from build123d import *

# Parameters (mm, degrees)
F1_DEPTH = 25.4
F2_R     = 28.1548982212
F3_DEPTH = 25.401
F4_R     = 12.69999


# Not quite as in the source:
# - a fillet or chamfer is up to 0.001 mm smaller than in the source, because OpenCascade refuses the exact size


with BuildPart() as f1:
    # F0 (on Front) → F1 (new body)
    with BuildSketch(Plane.XZ):
        Polygon((0, 63.7160863788), (0, 0), (254, 0), (254, 177.8), (221.1352040053, 177.8), (221.1352040053, 63.7160863788), (125.8798138147, 63.7160863788), (125.8798138147, 177.8), align=None)
    extrude(amount=F1_DEPTH)

    # F2 (on face) → F3 (cut, through all)
    with BuildSketch(Plane(origin=(0, 0, 0), x_dir=(-1, 0, 0), z_dir=(0, 1, 0))):
        with Locations((-74.7735798359, 45.1450571418)):
            Circle(F2_R)
    extrude(amount=-F3_DEPTH, mode=Mode.SUBTRACT)

    # F4 (radius 12.7 in the source; OpenCascade refuses exactly that, so slightly less here)
    f4_edges = [f1.edges().sort_by_distance(p)[0] for p in [
        (102.928478, 0, 45.145057),
        (102.928478, -25.4, 45.145057),
    ]]
    fillet(f4_edges, radius=F4_R)


solid = f1.part
CAD build for the part. Positions are in the model's coordinates, mm. A direction names the side the tool comes from. Round coordinates to 2 decimals unless told otherwise and drop trailing zeros. Loops run counter-clockwise (first coordinate to the right, second up) from the corner with the lowest first, then second, coordinate; pieces in that order, holes last.
(1) Cut at A-A (z = 102). Give the cut face in (x, y).
(2) Drop flat-ended pins along their axis: pin 1 (1 mm diameter, centred on x = 129.5, y = -20.5, fed in from +Z); pin 2 (1 mm diameter, centred on y = -14, z = 149, fed in from -X); pin 3 (10 mm diameter, centred on x = 35, y = -16.5, fed in from +Z). Give the stop position or say it passes through.
(3) Two-plate mould, pull along X, no slides. Class faces 3 (the flat face through (254, -13, 88)), 4 (the flat face through (174, -13, 63.716)), 5 (the flat face through (125, 0, 70)), 6 (the flat face through (221.135, -13, 122)): +X half, -X half, draft (parallel to the pull), parting line (faces both ways), or undercut.
(4) Cut at D-D (z = 127). Give the cut face in (x, y).
(5) Wall check: line 1 along X through (y, z) = (-4, 72.5); line 2 along Z through (x, y) = (215, -1.5); line 3 along X through (y, z) = (-18.5, 162). Give the ranges that are in metal, low to high.
(6) Cut at C-C (x = 200.5). Give the cut face in (y, z), plus the area to 3 significant figures.
(7) Cut at B-B (y = -7.25). Give the cut face in (x, z), plus the area to 3 significant figures.
(8) Which spindle directions (+Z, -Z, +X, -X, +Y, -Y) get a long thin tool onto all of the face, cutting with end or side? Do faces 1 (the flat face through (125.88, -13, 120)), 2 (the flat face through (63.821, -12.522, 121.557)). Say none if no direction does.
Findings below:
1. outline: (42.24, -25.4) - (125.88, -25.4) - (125.88, 0) - (42.24, 0) - close; (221.14, -25.4) - (254, -25.4) - (254, 0) - (221.14, 0) - close
2. pin 1: stops at z = 63.72
2. pin 2: stops at x = 93.55
2. pin 3: stops at z = 99.97
3. face 3: +X half
3. face 4: undercut
3. face 5: draft
3. face 6: undercut
4. outline: (69.83, -25.4) - (125.88, -25.4) - (125.88, 0) - (69.83, 0) - close; (221.14, -25.4) - (254, -25.4) - (254, 0) - (221.14, 0) - close
5. line 1: x = 9.69 to 58.95, 90.6 to 125.88, 221.14 to 254
5. line 2: z = 0 to 63.72
5. line 3: x = 108.45 to 125.88, 221.14 to 254
6. outline: (-25.4, 0) - (0, 0) - (0, 63.72) - (-25.4, 63.72) - close
6. area: 1,620 mm2
7. outline: (0, 0) - (254, 0) - (254, 177.8) - (221.14, 177.8) - (221.14, 63.72) - (125.88, 63.72) - (125.88, 177.8) - (0, 63.72) - close; hole circle Ø58.77 at (74.77, 45.15)
7. area: 24,400 mm2
8. face 1: +Z, +Y, -Y
8. face 2: +Z, -X, +Y, -Y
